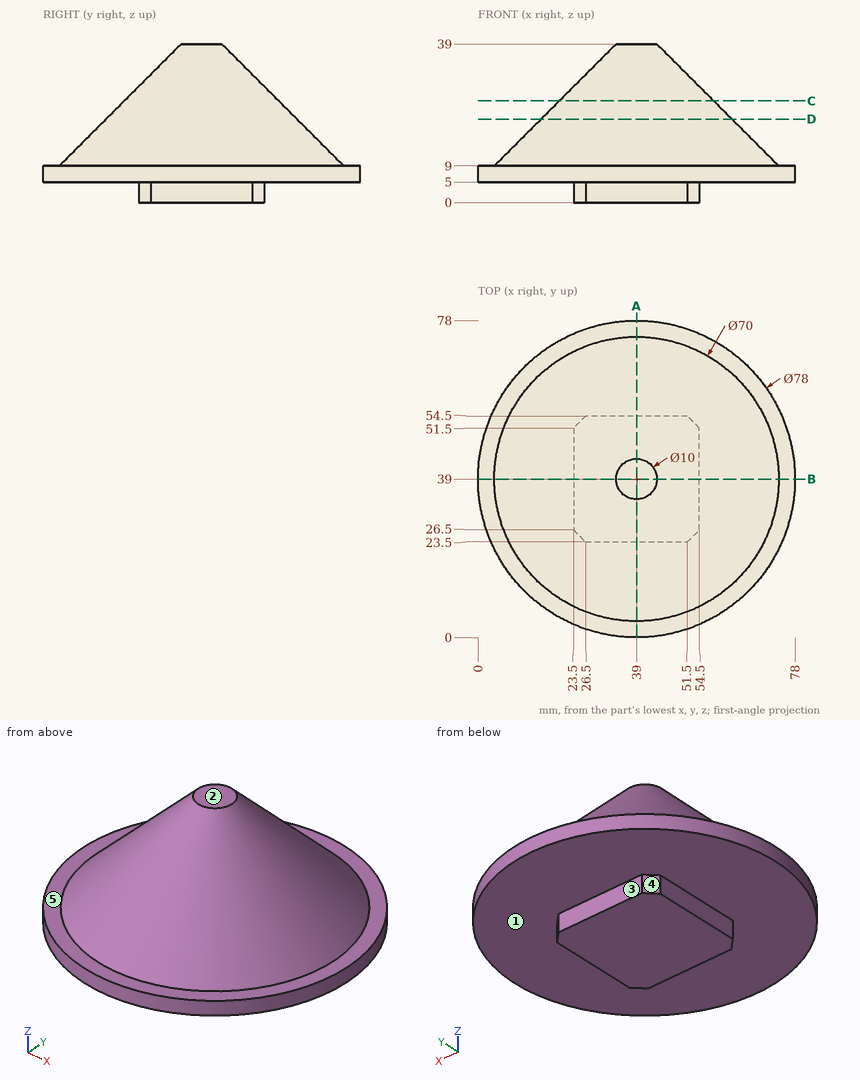
Design review of the part shown in the three views and the two pictorial views. Dimensions are in mm from the part's minimum x, y and z. A direction names the side the tool comes from. Round coordinates to 2 decimals unless told otherwise and drop trailing zeros. Write each loop counter-clockwise with the first axis right and the second up, starting at its lowest first coordinate (ties: lowest second). Pieces come first, ordered by that corner, then holes. Notation, with made-up numbers: M 51,81.25 L 90,81.25 A26 ccw 90,101.25 Z; hole C -7,89 d2. An arc over 180 degrees is marked long. One line per item, written item: value. Start each with the question number.
1. Clearance check with flat-ended pins moving along their axes: P1, Ø8, axis at x = 20, y = 17, coming from the +Z side; P2, Ø5, axis at x = 23.5, z = 8, coming from the -Y side; P3, Ø10, axis at y = 14.5, z = 12, coming from the -X side. State where each tip first meets the part, or that it passes through.
2. Take a section at A-A on x = 39. State the section outline as (y, z) points.
3. Take a section at C-C on z = 25. State the section outline as (x, y) points, then the cut area to 3 significant figures.
4. Take a section at D-D on z = 20.5. State the section outline as (x, y) points, then the cut area to 3 significant figures.
5. To check wall thickness, follow probe 1 along Z at (x, y) = (72, 58.5); probe 2 along Z at (x, y) = (10, 42); probe 3 along Y at (x, z) = (43, 25.5). State the ranges of each line that lie inside material, in increasing order. Write a range as from..to.
6. For the marked faces 1, 2, 3, 4 and 5, list the 3-axis set-ups (+Z, -Z, +X, -X, +Y, -Y) from which the entire face can be reached by the end or side of a thin tool; tool diameter is ignored.
Computed:
1. P1: stops at z = 18.93
1. P2: stops at y = 2.23
1. P3: stops at x = 5.82
2. outline: M 0,5 L 23.5,5 L 23.5,0 L 54.5,0 L 54.5,5 L 78,5 L 78,9 L 74,9 L 44,39 L 34,39 L 4,9 L 0,9 Z
3. outline: C 39,39 d38
3. area: 1,130 mm²
4. outline: C 39,39 d47
4. area: 1,730 mm²
5. probe 1: z = 5..9
5. probe 2: z = 5..14.85
5. probe 3: y = 20.94..57.06
6. face 1: -Z
6. face 2: +Z, +X, -X, +Y, -Y
6. face 3: -Z, +X, -X, +Y
6. face 4: -Z, -X, +Y
6. face 5: +Z
